from build123d import *

# Parameters (mm, degrees)
SKETCH_1_R               = 3
SKETCH_1_R_2             = 1.40625
EXTRUDE_1_DEPTH          = 5
CUT_EXTRUDE_2_DEPTH      = 7.557438524
PATTERN_CIRCULAR_1_COUNT = 7
SKETCH_2_R               = 3
EXTRUDE_2_DEPTH          = 4.8
CUT_EXTRUDE_START        = 4.8
CUT_EXTRUDE_3_DEPTH      = 3.8


with BuildPart() as part:
    # 草图1 → 凸台-拉伸1 (new body)
    with BuildSketch(Plane.XY):
        Circle(SKETCH_1_R)
        Circle(SKETCH_1_R_2, mode=Mode.SUBTRACT)
    extrude(amount=EXTRUDE_1_DEPTH)

    # 草图1<3> → 切除-拉伸2 (cut, through all)
    with BuildSketch(Plane.XY):
        with BuildLine():
            Line((1.546319716, 0.559598866), (1.322324253, 0.478536971))
            ThreePointArc((1.322324253, 0.478536971), (1.385109661, 0.242920339), (1.40625, 0))
            ThreePointArc((1.40625, 0), (1.385109661, -0.242920339), (1.322324253, -0.478536971))
            Line((1.322324253, -0.478536971), (1.546319716, -0.559598866))
            add(Edge.make_bspline(
                [(1.546319716, -0.559598866), (1.558105463, -0.563864019), (1.591921474, -0.573215837), (1.658734166, -0.580959295), (1.767731952, -0.57845396), (1.907008009, -0.553308364), (2.079413065, -0.496026363), (2.261035814, -0.40341458), (2.393734523, -0.311147352), (2.48335867, -0.236539754), (2.523284743, -0.200650618)],
                knots=[0, 0, 0, 0, 0, 0.005604068, 0.015718248, 0.029959916, 0.048733667, 0.068727063, 0.096888892, 0.120945025, 0.120945025, 0.120945025, 0.120945025, 0.120945025], degree=4))
            ThreePointArc((2.523284743, -0.200650618), (2.529257902, -0.100404327), (2.53125, 0))
            ThreePointArc((2.53125, 0), (2.529257902, 0.100404327), (2.523284743, 0.200650618))
            add(Edge.make_bspline(
                [(1.546319716, 0.559598866), (1.558105463, 0.563864019), (1.591921474, 0.573215837), (1.658734166, 0.580959295), (1.767731952, 0.57845396), (1.907008009, 0.553308364), (2.079413065, 0.496026363), (2.261035814, 0.40341458), (2.393734523, 0.311147352), (2.48335867, 0.236539754), (2.523284743, 0.200650618)],
                knots=[0, 0, 0, 0, 0, 0.005604068, 0.015718248, 0.029959916, 0.048733667, 0.068727063, 0.096888892, 0.120945025, 0.120945025, 0.120945025, 0.120945025, 0.120945025], degree=4))
        make_face()
    cut_extrude_2 = extrude(amount=CUT_EXTRUDE_2_DEPTH, mode=Mode.SUBTRACT)

    # 阵列(圆周)1: 切除-拉伸2 ×7 about axis
    pattern_circular_1_axis = Axis((0, 0, 5), (0, 0, 1))
    for i in range(1, PATTERN_CIRCULAR_1_COUNT):
        add(cut_extrude_2.rotate(pattern_circular_1_axis, i * 360 / PATTERN_CIRCULAR_1_COUNT), mode=Mode.SUBTRACT)

    # 草图2 → 凸台-拉伸2 (add)
    with BuildSketch(Plane.XY.offset(5)):
        Circle(SKETCH_2_R)
    extrude(amount=EXTRUDE_2_DEPTH)

    # 草图2<4> → 切除-拉伸3 (cut)
    with BuildSketch(Plane.XY.offset(5).offset(CUT_EXTRUDE_START)):
        with BuildLine():
            ThreePointArc((1.130029762, 2.230029762), (0, 2.5), (-1.130029762, 2.230029762))
            Line((-1.130029762, 2.230029762), (-1.130029762, 1.130029762))
            Line((-1.130029762, 1.130029762), (-2.230029762, 1.130029762))
            ThreePointArc((-2.230029762, 1.130029762), (-2.5, 0), (-2.230029762, -1.130029762))
            Line((-2.230029762, -1.130029762), (-1.130029762, -1.130029762))
            Line((-1.130029762, -1.130029762), (-1.130029762, -2.230029762))
            ThreePointArc((-1.130029762, -2.230029762), (0, -2.5), (1.130029762, -2.230029762))
            Line((1.130029762, -2.230029762), (1.130029762, -1.130029762))
            Line((1.130029762, -1.130029762), (2.230029762, -1.130029762))
            ThreePointArc((2.230029762, -1.130029762), (2.5, 0), (2.230029762, 1.130029762))
            Line((2.230029762, 1.130029762), (1.130029762, 1.130029762))
            Line((1.130029762, 1.130029762), (1.130029762, 2.230029762))
        make_face()
    extrude(amount=-CUT_EXTRUDE_3_DEPTH, mode=Mode.SUBTRACT)


solid = part.part
For this review, take the finished solid that the model builds, in its own axes (mm). A direction names the side the tool comes from. Round coordinates to 2 decimals unless told otherwise and drop trailing zeros. Write each loop counter-clockwise with the first axis right and the second up, starting at its lowest first coordinate (ties: lowest second). Pieces come first, ordered by that corner, then holes. Notation, with made-up numbers: M 44.25,-26 L 58.25,-26 A29 ccw 58.25,6 Z; hole C -12,-22 d4. An arc over 180 degrees is marked long. Write item = value, one per line. Start each with the question number.
(1) For line 1 along X through (y, z) = (-1.75, 1.5); line 2 along Z through (x, y) = (1, 1.5); line 3 along Y through (x, z) = (-1.25, 1.25), list the stretches that pass through material, from the lowest coordinate up.
(2) We need section A-A (z = 9.25). Give the boundary of the cut face in (x, y).
(3) Clearance check with flat-ended pins moving along their axes: pin 1 Ø0.6 at (x, z) = (1.5, 8) entering from +Y; pin 2 Ø1.2 at (x, z) = (2, 7.5) entering from -Y; pin 3 Ø1.2 at (y, z) = (2, 8) entering from +X. State where each tip first meets the part, or that it passes through.
(4) The part is to be moulded in two halves that separate along Y. For faces 1 (the face through (1.3, -1.3, 9.8)), 2 (the face through (-3, 0, 5)), 3 (the face through (1.13, 2, 8)), say which applies: +Y half, -Y half, draft (parallel to the pull), parting line (faces both ways), or undercut.
(5) For faces 4 (the face through (2, -1, 0)), 5 (the face through (-1.13, -2, 8)), list the 3-axis set-ups (+Z, -Z, +X, -X, +Y, -Y) from which the entire face can be reached by the end or side of a thin tool; tool diameter is ignored.
Results found:
q1.line_1 = -2.44 to -0.96, 0.19 to 0.66, 1.73 to 2.44
q1.line_2 = 5 to 6
q1.line_3 = -2.73 to -1.24, 1.24 to 2.73
q2.outline = C 0,0 d6; hole M -2.23,-1.13 L -1.13,-1.13 L -1.13,-2.23 A2.5 ccw 1.13,-2.23 L 1.13,-1.13 L 2.23,-1.13 A2.5 ccw 2.23,1.13 L 1.13,1.13 L 1.13,2.23 A2.5 ccw -1.13,2.23 L -1.13,1.13 L -2.23,1.13 A2.5 ccw Z
q3.pin_1 = 2.75
q3.pin_2 = -2.65
q3.pin_3 = 2.65
q4.face_1 = draft
q4.face_2 = parting line
q4.face_3 = undercut
q5.face_4 = -Z, +X, -X, +Y, -Y
q5.face_5 = +Z
